```python
from build123d import *

# Parameters (mm, degrees)
SKETCH_1_W          = 80
SKETCH_1_H          = 52
EXTRUDE_1_DEPTH     = 5
SKETCH_2_R          = 7
CUT_EXTRUDE_1_DEPTH = 5
CUT_EXTRUDE_3_DEPTH = 10
SKETCH_7_R          = 5
CUT_EXTRUDE_4_DEPTH = 10
SKETCH_10_W         = 10
SKETCH_10_H         = 5
CUT_EXTRUDE_5_DEPTH = 10
SKETCH_11_R         = 1
CUT_EXTRUDE_6_DEPTH = 10
SKETCH_12_W         = 5
SKETCH_12_H         = 6.9
EXTRUDE_3_DEPTH     = 5
SKETCH_13_R         = 1
CUT_EXTRUDE_7_DEPTH = 5
FILLET_1_R          = 1
SKETCH_14_W         = 20
SKETCH_14_H         = 5
EXTRUDE_4_DEPTH     = 5
FILLET_2_R          = 1


with BuildPart() as part:
    # 스케치1 → 보스-돌출1 (new body)
    with BuildSketch(Plane.XY):
        with Locations((40, 26)):
            Rectangle(SKETCH_1_W, SKETCH_1_H)
    extrude(amount=EXTRUDE_1_DEPTH)

    # 스케치2 → 컷-돌출1 (cut)
    with BuildSketch(Plane.XY.offset(5)):
        with Locations((71.393420887, 43.125)):
            Circle(SKETCH_2_R)
    extrude(amount=-CUT_EXTRUDE_1_DEPTH, mode=Mode.SUBTRACT)

    # 스케치6 → 컷-돌출3 (cut)
    with BuildSketch(Plane.XY.offset(5)):
        with BuildLine():
            Line((0, 31.55), (6, 31.55))
            Line((6, 31.55), (6, 32.75))
            ThreePointArc((6, 32.75), (7.4, 34.15), (8.8, 32.75))
            Line((8.8, 32.75), (8.8, 31.55))
            Line((8.8, 31.55), (10, 31.55))
            ThreePointArc((10, 31.55), (11.55, 30), (10, 28.45))
            Line((10, 28.45), (8.8, 28.45))
            Line((8.8, 28.45), (8.8, 27.25))
            ThreePointArc((8.8, 27.25), (7.4, 25.85), (6, 27.25))
            Line((6, 27.25), (6, 28.45))
            Line((6, 28.45), (0, 28.45))
            Line((0, 28.45), (0, 31.55))
        make_face()
        with BuildLine():
            Line((0, 11.55), (6, 11.55))
            Line((6, 11.55), (6, 12.75))
            ThreePointArc((6, 12.75), (7.4, 14.15), (8.8, 12.75))
            Line((8.8, 12.75), (8.8, 11.55))
            Line((8.8, 11.55), (10, 11.55))
            ThreePointArc((10, 11.55), (11.55, 10), (10, 8.45))
            Line((10, 8.45), (8.8, 8.45))
            Line((8.8, 8.45), (8.8, 7.25))
            ThreePointArc((8.8, 7.25), (7.4, 5.85), (6, 7.25))
            Line((6, 7.25), (6, 8.45))
            Line((6, 8.45), (0, 8.45))
            Line((0, 8.45), (0, 11.55))
        make_face()
        with BuildLine():
            Line((74, 7.25), (74, 8.45))
            Line((74, 8.45), (80, 8.45))
            Line((80, 8.45), (80, 11.55))
            Line((80, 11.55), (74, 11.55))
            Line((74, 11.55), (74, 12.75))
            ThreePointArc((74, 12.75), (72.6, 14.15), (71.2, 12.75))
            Line((71.2, 12.75), (71.2, 11.55))
            Line((71.2, 11.55), (70, 11.55))
            ThreePointArc((70, 11.55), (68.45, 10), (70, 8.45))
            Line((70, 8.45), (71.2, 8.45))
            Line((71.2, 8.45), (71.2, 7.25))
            ThreePointArc((71.2, 7.25), (72.6, 5.85), (74, 7.25))
        make_face()
        with BuildLine():
            Line((74, 27.25), (74, 28.45))
            Line((74, 28.45), (80, 28.45))
            Line((80, 28.45), (80, 31.55))
            Line((80, 31.55), (74, 31.55))
            Line((74, 31.55), (74, 32.75))
            ThreePointArc((74, 32.75), (72.6, 34.15), (71.2, 32.75))
            Line((71.2, 32.75), (71.2, 31.55))
            Line((71.2, 31.55), (70, 31.55))
            ThreePointArc((70, 31.55), (68.45, 30), (70, 28.45))
            Line((70, 28.45), (71.2, 28.45))
            Line((71.2, 28.45), (71.2, 27.25))
            ThreePointArc((71.2, 27.25), (72.6, 25.85), (74, 27.25))
        make_face()
    extrude(amount=-CUT_EXTRUDE_3_DEPTH, mode=Mode.SUBTRACT)

    # 스케치7 → 컷-돌출4 (cut)
    with BuildSketch(Plane.XY.offset(5)):
        with Locations((32.75, 37.557368355)):
            Circle(SKETCH_7_R)
        with Locations((47.25, 12.442631645)):
            Circle(SKETCH_7_R)
    extrude(amount=-CUT_EXTRUDE_4_DEPTH, mode=Mode.SUBTRACT)

    # 스케치10 → 컷-돌출5 (cut)
    with BuildSketch(Plane(origin=(0, 0, 0), x_dir=(-1, 0, 0), z_dir=(0, 0, -1))):
        with Locations((-25, 2.5)):
            Rectangle(SKETCH_10_W, SKETCH_10_H)
        with Locations((-55, 2.5)):
            Rectangle(SKETCH_10_W, SKETCH_10_H)
    extrude(amount=-CUT_EXTRUDE_5_DEPTH, mode=Mode.SUBTRACT)

    # 스케치11 → 컷-돌출6 (cut)
    with BuildSketch(Plane.XY.offset(5)):
        with Locations((59, 5)):
            Circle(SKETCH_11_R)
        with Locations((51, 5)):
            Circle(SKETCH_11_R)
        with Locations((29, 5)):
            Circle(SKETCH_11_R)
        with Locations((21, 5)):
            Circle(SKETCH_11_R)
    extrude(amount=-CUT_EXTRUDE_6_DEPTH, mode=Mode.SUBTRACT)

    # 스케치12 → 보스-돌출3 (add)
    with BuildSketch(Plane.XY.offset(5)):
        with Locations((82.5, 20)):
            Rectangle(SKETCH_12_W, SKETCH_12_H)
        with Locations((-2.5, 20)):
            Rectangle(SKETCH_12_W, SKETCH_12_H)
    extrude(amount=-EXTRUDE_3_DEPTH)

    # 스케치13 → 컷-돌출7 (cut)
    with BuildSketch(Plane.XY.offset(5)):
        with Locations((80, 24.45)):
            Circle(SKETCH_13_R)
        with Locations((80, 15.55)):
            Circle(SKETCH_13_R)
        with Locations((0, 15.55)):
            Circle(SKETCH_13_R)
        with Locations((0, 24.45)):
            Circle(SKETCH_13_R)
    extrude(amount=-CUT_EXTRUDE_7_DEPTH, mode=Mode.SUBTRACT)

    # 필렛1
    fillet_1_edges = [part.edges().sort_by_distance(p)[0] for p in [
        (85, 23.45, 2.5),
        (85, 16.55, 2.5),
        (-5, 16.55, 2.5),
        (-5, 23.45, 2.5),
    ]]
    fillet(fillet_1_edges, radius=FILLET_1_R)

    # 스케치14 → 보스-돌출4 (add)
    with BuildSketch(Plane.XY.offset(5)):
        with Locations((70, -2.5)):
            Rectangle(SKETCH_14_W, SKETCH_14_H)
        with Locations((10, -2.5)):
            Rectangle(SKETCH_14_W, SKETCH_14_H)
    extrude(amount=-EXTRUDE_4_DEPTH)

    # 필렛2
    fillet_2_edges = [part.edges().sort_by_distance(p)[0] for p in [
        (80, -5, 2.5),
        (60, -5, 2.5),
        (0, -5, 2.5),
        (20, -5, 2.5),
    ]]
    fillet(fillet_2_edges, radius=FILLET_2_R)


solid = part.part
```
Model file for the job. Use its own axes, mm. A direction names the side the tool comes from. Coordinates: 2 decimals unless noted, no trailing zeros. Loops run counter-clockwise (first coordinate to the right, second up) from the corner with the lowest first, then second, coordinate; pieces in that order, holes last. Notation, with made-up numbers: M -26.5,81.5 L 7.5,81.5 A21 ccw 7.5,120.5 Z; hole C 74.25,83.5 d4. An arc over 180 degrees is marked long. Use CSV: the item, a comma, the result in double quotes. Start each with the question number.
1. Band-saw the part on D-D, the plane y = 24.45. List the corners of the cut face in (x, z), then the cut area to 3 significant figures.
2. Two-plate mould, pull along Y, no slides. Class faces 5 (the cylindrical face through (31.666, 32.676, 2.535)), 6 (the flat face through (20, 0, 2)), 7 (the cylindrical face through (21, 6, 3)), 8 (the cylindrical face through (79, 24.5, 2.5)): pulls with the +Y half, pulls with the -Y half, needs draft (parallel to the pull), parting line crosses it, or undercut.
3. Flat gauge pins, fed straight in: pin 1 (0.6 mm diameter, centred on y = 12, z = 2, fed in from -X); pin 2 (8 mm diameter, centred on x = 47.25, y = 12.44, fed in from +Z); pin 3 (1 mm diameter, centred on y = 12.5, z = 3, fed in from +X). Where does each tip first touch, or does it go through?
4. Band-saw the part on B-B, the plane y = 10. List the corners of the cut face in (x, z), then the cut area to 3 significant figures.
5. Tool access for faces 1 (the flat face through (0, 27, 2)), 2 (the flat face through (55, 5, 2)), 3 (the flat face through (77, 28.45, 3)), 4 (the cylindrical face through (72.57, 5.85, 2.54)): list every direction of +Z, -Z, +X, -X, +Y, -Y with a clear straight run to the whole face (end or side of a thin tool).
6. Probe probe 1 along X at (y, z) = (12, 2.75); probe 2 along X at (y, z) = (3, 4); probe 3 along X at (y, z) = (43, 3.6). List the from-to ranges inside material, lowest first. Write a range as [from, to].
7. Band-saw the part on C-C, the plane x = 23.5. List the corners of the cut face in (y, z).
8. Band-saw the part on A-A, the plane x = 47.25. List the corners of the cut face in (y, z).
Entries:
1,outline,"M 1,0 L 79,0 L 79,5 L 1,5 Z"
1,area,"390 mm2"
2,face 5,"undercut"
2,face 6,"needs draft"
2,face 7,"pulls with the -Y half"
2,face 8,"undercut"
3,pin 1,"stops at x = 0"
3,pin 2,"passes through"
3,pin 3,"stops at x = 80"
4,outline,"M 11.55,0 L 42.89,0 L 42.89,5 L 11.55,5 Z; M 51.61,0 L 68.45,0 L 68.45,5 L 51.61,5 Z"
4,area,"241 mm2"
5,face 1,"+Z, -Z, -X, +Y"
5,face 2,"+Z, -Z, -Y"
5,face 3,"+Z, -Z, +X"
5,face 4,"+Z, -Z"
6,probe 1,"x = [0, 6], [8.8, 42.27], [52.23, 71.2], [74, 80]"
6,probe 2,"x = [0, 20], [30, 50], [60, 80]"
6,probe 3,"x = [0, 64.39], [78.39, 80]"
7,outline,"M 5,0 L 52,0 L 52,5 L 5,5 Z"
8,outline,"M 0,0 L 7.44,0 L 7.44,5 L 0,5 Z; M 17.44,0 L 52,0 L 52,5 L 17.44,5 Z"
